```python
from build123d import *

# Parameters (mm, degrees)
SKETCH1_W           = 16
SKETCH1_H           = 4
BOSS_EXTRUDE1_DEPTH = 1.5
SKETCH2_W           = 0.5
SKETCH2_H           = 0.5
CUT_EXTRUDE1_DEPTH  = 2


with BuildPart() as part:
    # Sketch1 → Boss-Extrude1 (new body)
    with BuildSketch(Plane(origin=(0, 0, 0), x_dir=(1, 0, 0), z_dir=(0, 1, 0))):
        with Locations((8, 2)):
            Rectangle(SKETCH1_W, SKETCH1_H)
    extrude(amount=BOSS_EXTRUDE1_DEPTH)

    # Sketch2 → Cut-Extrude1 (cut)
    with BuildSketch(Plane(origin=(0, 1.5, 0), x_dir=(1, 0, 0), z_dir=(0, 1, 0))):
        with Locations((3, 3)):
            Rectangle(SKETCH2_W, SKETCH2_H)
        with Locations((1, 3)):
            Rectangle(SKETCH2_W, SKETCH2_H)
        with Locations((5, 3)):
            Rectangle(SKETCH2_W, SKETCH2_H)
        with Locations((7, 3)):
            Rectangle(SKETCH2_W, SKETCH2_H)
        with Locations((9, 3)):
            Rectangle(SKETCH2_W, SKETCH2_H)
        with Locations((11, 3)):
            Rectangle(SKETCH2_W, SKETCH2_H)
        with Locations((13, 3)):
            Rectangle(SKETCH2_W, SKETCH2_H)
        with Locations((15, 3)):
            Rectangle(SKETCH2_W, SKETCH2_H)
        with Locations((17, 3)):
            Rectangle(SKETCH2_W, SKETCH2_H)
        with Locations((19, 3)):
            Rectangle(SKETCH2_W, SKETCH2_H)
        with Locations((21, 3)):
            Rectangle(SKETCH2_W, SKETCH2_H)
        with Locations((23, 3)):
            Rectangle(SKETCH2_W, SKETCH2_H)
        with Locations((25, 3)):
            Rectangle(SKETCH2_W, SKETCH2_H)
        with Locations((27, 3)):
            Rectangle(SKETCH2_W, SKETCH2_H)
        with Locations((29, 3)):
            Rectangle(SKETCH2_W, SKETCH2_H)
        with Locations((31, 3)):
            Rectangle(SKETCH2_W, SKETCH2_H)
        with Locations((33, 3)):
            Rectangle(SKETCH2_W, SKETCH2_H)
        with Locations((35, 3)):
            Rectangle(SKETCH2_W, SKETCH2_H)
        with Locations((1, 1)):
            Rectangle(SKETCH2_W, SKETCH2_H)
        with Locations((3, 1)):
            Rectangle(SKETCH2_W, SKETCH2_H)
        with Locations((5, 1)):
            Rectangle(SKETCH2_W, SKETCH2_H)
        with Locations((7, 1)):
            Rectangle(SKETCH2_W, SKETCH2_H)
        with Locations((9, 1)):
            Rectangle(SKETCH2_W, SKETCH2_H)
        with Locations((11, 1)):
            Rectangle(SKETCH2_W, SKETCH2_H)
        with Locations((13, 1)):
            Rectangle(SKETCH2_W, SKETCH2_H)
        with Locations((15, 1)):
            Rectangle(SKETCH2_W, SKETCH2_H)
        with Locations((17, 1)):
            Rectangle(SKETCH2_W, SKETCH2_H)
        with Locations((19, 1)):
            Rectangle(SKETCH2_W, SKETCH2_H)
        with Locations((21, 1)):
            Rectangle(SKETCH2_W, SKETCH2_H)
        with Locations((23, 1)):
            Rectangle(SKETCH2_W, SKETCH2_H)
        with Locations((25, 1)):
            Rectangle(SKETCH2_W, SKETCH2_H)
        with Locations((27, 1)):
            Rectangle(SKETCH2_W, SKETCH2_H)
        with Locations((29, 1)):
            Rectangle(SKETCH2_W, SKETCH2_H)
        with Locations((31, 1)):
            Rectangle(SKETCH2_W, SKETCH2_H)
        with Locations((33, 1)):
            Rectangle(SKETCH2_W, SKETCH2_H)
        with Locations((35, 1)):
            Rectangle(SKETCH2_W, SKETCH2_H)
    extrude(amount=-CUT_EXTRUDE1_DEPTH, mode=Mode.SUBTRACT)


solid = part.part
```
Design review of the part built by this model. Coordinates are the model's own, in mm. Give positions to 0.01 mm unless a question says otherwise; leave off trailing zeros. Write each loop counter-clockwise with the first axis right and the second up, starting at its lowest first coordinate (ties: lowest second). Pieces come first, ordered by that corner, then holes.
(1) Clearance check with a flat-ended pin moving along its axis: pin 1 Ø0.6 at (y, z) = (0.5, -3) entering from -X. State where the tip first meets the part, or that it passes through.
Checked values:
pin 1: stops at x = 0
(2) Add section B-B (z = -1.1). Give the number of separate pieces and of enclosed holes in the cut face, and give its area (3 significant figures).
Checked values:
separate pieces: 9
enclosed holes: 0
area: 18.0 mm2
(3) Wall thickness on line 1 along Z through (x, y) = (13, 1.3): over which ranges is the line inside the solid? List them lowest first.
Checked values:
line 1: z = -4 to -3.25, -2.75 to -1.25, -0.75 to 0
(4) Add section A-A (x = 5). Give the boundary of the cut face in (y, z), and give its area (3 significant figures).
Checked values:
outline: (0, -4) - (1.5, -4) - (1.5, -3.25) - (0, -3.25) - close; (0, -2.75) - (1.5, -2.75) - (1.5, -1.25) - (0, -1.25) - close; (0, -0.75) - (1.5, -0.75) - (1.5, 0) - (0, 0) - close
area: 4.50 mm2
